Geometry check sheet. Reference: the model listing, model coordinates, mm. Coordinates: 2 decimals unless noted, no trailing zeros. Write each loop counter-clockwise with the first axis right and the second up, starting at its lowest first coordinate (ties: lowest second). Pieces come first, ordered by that corner, then holes. Notation, with made-up numbers: M -11,86 L 17,86 A15 ccw 17,115 Z; hole C 62.25,32.5 d1. An arc over 180 degrees is marked long. Answer as a JSON object with one key per item and string values. Group by question number.
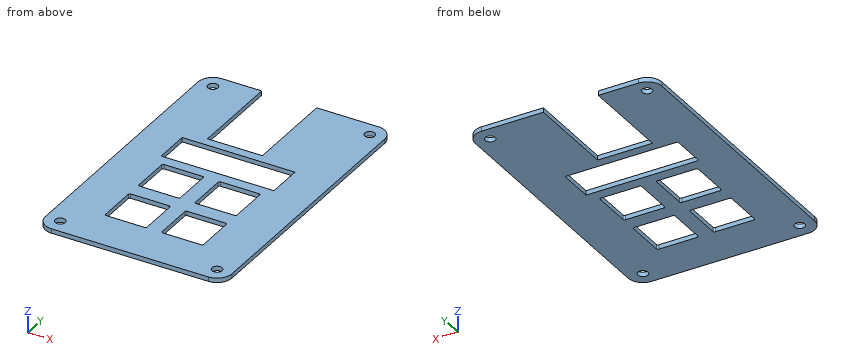
Autodesk Fusion 360 part; units mm, degrees
sketch "plate-2025-11-24T01_24_03.301Z" plane through (0, 0, 0) normal (0, 0, 1) x (1, 0, 0)
  line L0 (3.025, -2.525) -> (16.025, -2.525)
  line L1 (3.025, -16.525) -> (16.025, -16.525)
  line L2 (2.525, -3.025) -> (2.525, -16.025)
  line L3 (16.525, -3.025) -> (16.525, -16.025)
  arc A0 (3.025, -2.525) -> (2.525, -3.025) centre (3.025, -3.025) ccw
  arc A1 (16.525, -3.025) -> (16.025, -2.525) centre (16.025, -3.025) ccw
  arc A2 (2.525, -16.025) -> (3.025, -16.525) centre (3.025, -16.025) ccw
  arc A3 (16.025, -16.525) -> (16.525, -16.025) centre (16.025, -16.025) ccw
  line L4 (22.075, -2.525) -> (35.075, -2.525)
  line L5 (22.075, -16.525) -> (35.075, -16.525)
  line L6 (21.575, -3.025) -> (21.575, -16.025)
  line L7 (35.575, -3.025) -> (35.575, -16.025)
  arc A4 (22.075, -2.525) -> (21.575, -3.025) centre (22.075, -3.025) ccw
  arc A5 (35.575, -3.025) -> (35.075, -2.525) centre (35.075, -3.025) ccw
  arc A6 (21.575, -16.025) -> (22.075, -16.525) centre (22.075, -16.025) ccw
  arc A7 (35.075, -16.525) -> (35.575, -16.025) centre (35.075, -16.025) ccw
  line L8 (3.025, -21.575) -> (16.025, -21.575)
  line L9 (3.025, -35.575) -> (16.025, -35.575)
  line L10 (2.525, -22.075) -> (2.525, -35.075)
  line L11 (16.525, -22.075) -> (16.525, -35.075)
  arc A8 (3.025, -21.575) -> (2.525, -22.075) centre (3.025, -22.075) ccw
  arc A9 (16.525, -22.075) -> (16.025, -21.575) centre (16.025, -22.075) ccw
  arc A10 (2.525, -35.075) -> (3.025, -35.575) centre (3.025, -35.075) ccw
  arc A11 (16.025, -35.575) -> (16.525, -35.075) centre (16.025, -35.075) ccw
  line L12 (22.075, -21.575) -> (35.075, -21.575)
  line L13 (22.075, -35.575) -> (35.075, -35.575)
  line L14 (21.575, -22.075) -> (21.575, -35.075)
  line L15 (35.575, -22.075) -> (35.575, -35.075)
  arc A12 (22.075, -21.575) -> (21.575, -22.075) centre (22.075, -22.075) ccw
  arc A13 (35.575, -22.075) -> (35.075, -21.575) centre (35.075, -22.075) ccw
  arc A14 (21.575, -35.075) -> (22.075, -35.575) centre (22.075, -35.075) ccw
  arc A15 (35.075, -35.575) -> (35.575, -35.075) centre (35.075, -35.075) ccw
sketch "Sketch2" plane through (0, 0, 0) normal (0, 0, 1) x (1, 0, 0)
  line L0 (-11.896, 47.235) -> (50.966, 47.235)
  line L1 (50.966, 47.235) -> (50.966, -49.996)
  line L2 (50.966, -49.996) -> (-11.896, -49.996)
  line L3 (-11.896, -49.996) -> (-11.896, 47.235)
  line L4 (2.525, -22.075) -> (2.525, -35.075)
  line L5 (3.025, -35.575) -> (16.025, -35.575)
  circle A0 centre (-6.896, 42.235) radius 1.7
  circle A1 centre (45.966, 42.235) radius 1.7
  circle A2 centre (45.966, -44.996) radius 1.7
  circle A3 centre (-6.896, -44.996) radius 1.7
  line L6 (6.603, 47.235) -> (25.103, 47.235)
  line L7 (25.103, 47.235) -> (25.103, 16.235)
  line L8 (25.103, 16.235) -> (6.603, 16.235)
  line L9 (6.603, 16.235) -> (6.603, 47.235)
  dimension "d1" = 62.862
  dimension "d2" = 97.231
  dimension "d3" = 14.421
  dimension "d4" = 14.421
  dimension "d8" = 3.4
  dimension "d9" = 5
  dimension "d10" = 5
  dimension "d11" = 3.4
  dimension "d12" = 5
  dimension "d13" = 5
  dimension "d14" = 3.4
  dimension "d15" = 5
  dimension "d16" = 5
  dimension "d17" = 3.4
  dimension "d18" = 5
  dimension "d19" = 5
  dimension "d20" = 18.5
  dimension "d21" = 31
  dimension "d22" = 18.499
extrude "Extrude1" add sketch "Sketch2" along normal blind 1.5 contours L0 L1 L2 L3 L7 L8 L9
extrude "Extrude2" cut sketch "plate-2025-11-24T01_24_03.301Z" along normal blind 1.5
fillet "Fillet1" radius 5 1 edges at (50.966, -49.996, 0.75)
fillet "Fillet2" radius 5 1 edges at (50.966, 47.235, 0.75)
fillet "Fillet3" radius 5 1 edges at (-11.896, 47.235, 0.75)
fillet "Fillet4" radius 5 1 edges at (-11.896, -49.996, 0.75)
sketch "Sketch3" plane through (0, 0, 1.5) normal (0, 0, 1) x (-1, 0, 0)
  arc A0 (11.896, 44.996) -> (6.896, 49.996) centre (6.896, 44.996) ccw
  line L0 (6.896, 49.996) -> (-45.966, 49.996)
  arc A1 (-45.966, 49.996) -> (-50.966, 44.996) centre (-45.966, 44.996) ccw
  line L1 (-50.966, 44.996) -> (-50.966, -42.235)
  arc A2 (-50.966, -42.235) -> (-45.966, -47.235) centre (-45.966, -42.235) ccw
  line L2 (-45.966, -47.235) -> (-25.103, -47.235)
  line L3 (-25.103, -47.235) -> (-25.103, -16.235)
  line L4 (-25.103, -16.235) -> (-6.603, -16.235)
  line L5 (-6.603, -16.235) -> (-6.603, -47.235)
  line L6 (-6.603, -47.235) -> (6.896, -47.235)
  arc A3 (6.896, -47.235) -> (11.896, -42.235) centre (6.896, -42.235) ccw
  line L7 (11.896, -42.235) -> (11.896, 44.996)
  line L8 (-22.075, 21.575) -> (-35.075, 21.575)
  arc A4 (-35.575, 22.075) -> (-35.075, 21.575) centre (-35.075, 22.075) ccw
  line L9 (-35.575, 22.075) -> (-35.575, 35.075)
  arc A5 (-35.075, 35.575) -> (-35.575, 35.075) centre (-35.075, 35.075) ccw
  line L10 (-35.075, 35.575) -> (-22.075, 35.575)
  arc A6 (-21.575, 35.075) -> (-22.075, 35.575) centre (-22.075, 35.075) ccw
  line L11 (-21.575, 35.075) -> (-21.575, 22.075)
  arc A7 (-22.075, 21.575) -> (-21.575, 22.075) centre (-22.075, 22.075) ccw
  line L12 (-3.025, 2.525) -> (-16.025, 2.525)
  arc A8 (-16.525, 3.025) -> (-16.025, 2.525) centre (-16.025, 3.025) ccw
  line L13 (-16.525, 3.025) -> (-16.525, 16.025)
  arc A9 (-16.025, 16.525) -> (-16.525, 16.025) centre (-16.025, 16.025) ccw
  line L14 (-16.025, 16.525) -> (-3.025, 16.525)
  arc A10 (-2.525, 16.025) -> (-3.025, 16.525) centre (-3.025, 16.025) ccw
  line L15 (-2.525, 16.025) -> (-2.525, 3.025)
  arc A11 (-3.025, 2.525) -> (-2.525, 3.025) centre (-3.025, 3.025) ccw
  line L16 (-3.025, 21.575) -> (-16.025, 21.575)
  arc A12 (-16.525, 22.075) -> (-16.025, 21.575) centre (-16.025, 22.075) ccw
  line L17 (-16.525, 22.075) -> (-16.525, 35.075)
  arc A13 (-16.025, 35.575) -> (-16.525, 35.075) centre (-16.025, 35.075) ccw
  line L18 (-16.025, 35.575) -> (-3.025, 35.575)
  arc A14 (-2.525, 35.075) -> (-3.025, 35.575) centre (-3.025, 35.075) ccw
  line L19 (-2.525, 35.075) -> (-2.525, 22.075)
  arc A15 (-3.025, 21.575) -> (-2.525, 22.075) centre (-3.025, 22.075) ccw
  line L20 (-22.075, 2.525) -> (-35.075, 2.525)
  arc A16 (-35.575, 3.025) -> (-35.075, 2.525) centre (-35.075, 3.025) ccw
  line L21 (-35.575, 3.025) -> (-35.575, 16.025)
  arc A17 (-35.075, 16.525) -> (-35.575, 16.025) centre (-35.075, 16.025) ccw
  line L22 (-35.075, 16.525) -> (-22.075, 16.525)
  arc A18 (-21.575, 16.025) -> (-22.075, 16.525) centre (-22.075, 16.025) ccw
  line L23 (-21.575, 16.025) -> (-21.575, 3.025)
  arc A19 (-22.075, 2.525) -> (-21.575, 3.025) centre (-22.075, 3.025) ccw
  circle A20 centre (6.896, -42.235) radius 1.7
  circle A21 centre (-45.966, 44.996) radius 1.7
  circle A22 centre (-45.966, -42.235) radius 1.7
  circle A23 centre (6.896, 44.996) radius 1.7
  line L24 (0.08, -13.128) -> (-37.92, -13.128)
  line L25 (-37.92, -13.128) -> (-37.92, -1.128)
  line L26 (-37.92, -1.128) -> (0.08, -1.128)
  line L27 (0.08, -1.128) -> (0.08, -13.128)
  line L28 (11.896, 49.996) -> (11.896, -47.235)
  dimension "d35" = 38
  dimension "d36" = 12
  dimension "d37" = 11.816
extrude "Extrude3" cut sketch "Sketch3" against normal blind 1.5 contours L24 L25 L26 L27
1) Section check C-C (y = 10.5). Record the cut outline in (x, z), then the cut area to 3 significant figures.
2) Section check D-D (z = 0.25). State how many separate pieces and enclosed holes the cut face has, then the cut area to 3 significant figures.
3) Go/stop test with a flat-tipped pin: pin 1 Ø2 at (x, y) = (45.966, 42.235) entering from +Z. Record where the tip stops, or that it passes through.
4) Section check A-A (x = 9). Record the cut outline in (y, z) (3 decimals).
5) Section check B-B (y = -31). Record the cut outline in (x, z) (3 decimals), then the cut area to 3 significant figures.
6) Material ranges on probe 1 along Y at (x, z) = (23, 0.1) (3 decimals); probe 2 along Y at (x, z) = (35, 1.35) (3 decimals); probe 3 along X at (y, z) = (-25, 0.35) (3 decimals), recorded low to high. Write a range as [from, to].
Entries:
{
 "1": {"outline": "M -11.9,0 L -0.08,0 L -0.08,1.5 L -11.9,1.5 Z; M 37.92,0 L 50.97,0 L 50.97,1.5 L 37.92,1.5 Z", "area": "37.3 mm^2"},
 "2": {"separate pieces": "1", "enclosed holes": "9", "area": "4,240 mm^2"},
 "3": {"pin 1": "through"},
 "4": {"outline": "M -49.996,0 L -35.575,0 L -35.575,1.5 L -49.996,1.5 Z; M -21.575,0 L -16.525,0 L -16.525,1.5 L -21.575,1.5 Z; M -2.525,0 L 1.128,0 L 1.128,1.5 L -2.525,1.5 Z; M 13.128,0 L 16.235,0 L 16.235,1.5 L 13.128,1.5 Z"},
 "5": {"outline": "M -11.896,0 L 2.525,0 L 2.525,1.5 L -11.896,1.5 Z; M 16.525,0 L 21.575,0 L 21.575,1.5 L 16.525,1.5 Z; M 35.575,0 L 50.966,0 L 50.966,1.5 L 35.575,1.5 Z", "area": "52.3 mm^2"},
 "6": {"probe 1": "[-49.996, -35.575], [-21.575, -16.525], [-2.525, 1.128], [13.128, 16.235]", "probe 2": "[-49.996, -35.575], [-21.575, -16.525], [-2.525, 1.128], [13.128, 47.235]", "probe 3": "[-11.896, 2.525], [16.525, 21.575], [35.575, 50.966]"}
}
